from build123d import *

# Parameters (mm, degrees)
IZIM1_W                     = 300
IZIM1_H                     = 120
Y_KSEKLIK_EKSTR_ZYON1_DEPTH = 20
IZIM2_W                     = 20
IZIM2_H                     = 120
Y_KSEKLIK_EKSTR_ZYON2_DEPTH = 70
IZIM3_W                     = 140
IZIM3_H                     = 120
Y_KSEKLIK_EKSTR_ZYON3_DEPTH = 20
Y_KSEKLIK_EKSTR_ZYON4_DEPTH = 20
AYNALAMA3_COPY_1_DEPTH      = 20
IZIM5_R                     = 35
KES_EKSTR_ZYON1_DEPTH       = 51
KES_EKSTR_ZYON1_DEPTH_BACK  = 41
IZIM6_R                     = 10
KES_EKSTR_ZYON2_DEPTH       = 20


with BuildPart() as part:
    # Çizim1 → Yükseklik-Ekstrüzyon1 (new body)
    with BuildSketch(Plane(origin=(0, 0, 0), x_dir=(1, 0, 0), z_dir=(0, 1, 0))):
        with Locations((150, 60)):
            Rectangle(IZIM1_W, IZIM1_H)
    extrude(amount=Y_KSEKLIK_EKSTR_ZYON1_DEPTH)

    # Çizim2 → Yükseklik-Ekstrüzyon2 (add)
    with BuildSketch(Plane(origin=(0, 20, 0), x_dir=(1, 0, 0), z_dir=(0, 1, 0))):
        with Locations((70, 60)):
            Rectangle(IZIM2_W, IZIM2_H)
    y_kseklik_ekstr_zyon2 = extrude(amount=Y_KSEKLIK_EKSTR_ZYON2_DEPTH)

    # Aynalama1: Yükseklik-Ekstrüzyon2 across plane
    add(y_kseklik_ekstr_zyon2.mirror(Plane.ZY.offset(-150)))

    # Çizim3 → Yükseklik-Ekstrüzyon3 (add)
    with BuildSketch(Plane(origin=(0, 20, 0), x_dir=(1, 0, 0), z_dir=(0, 1, 0))):
        with Locations((150, 60)):
            Rectangle(IZIM3_W, IZIM3_H)
    extrude(amount=Y_KSEKLIK_EKSTR_ZYON3_DEPTH)

    # Çizim4 → Yükseklik-Ekstrüzyon4 (add)
    with BuildSketch(Plane.XY):
        Polygon((0, 20), (60, 90), (60, 20), align=None)
    y_kseklik_ekstr_zyon4 = extrude(amount=-Y_KSEKLIK_EKSTR_ZYON4_DEPTH)

    # Aynalama2: Yükseklik-Ekstrüzyon4 across plane
    add(y_kseklik_ekstr_zyon4.mirror(Plane.XY.offset(-60)))

    # Aynalama3: Yükseklik-Ekstrüzyon4 across plane
    add(y_kseklik_ekstr_zyon4.mirror(Plane.ZY.offset(-150)))

    # Aynalama3 copy 1 sketch → Aynalama3 copy 1 (add)
    with BuildSketch(Plane(origin=(300, 0, -120), x_dir=(-1, 0, 0), z_dir=(0, 0, -1))):
        Polygon((0, 20), (60, 90), (60, 20), align=None)
    extrude(amount=-AYNALAMA3_COPY_1_DEPTH)

    # Çizim5 → Kes-Ekstrüzyon1 (cut, two sides)
    with BuildSketch(Plane(origin=(0, 40, 0), x_dir=(1, 0, 0), z_dir=(0, 1, 0))) as kes_ekstr_zyon1_sk:
        with Locations((150, 60)):
            Circle(IZIM5_R)
    extrude(amount=KES_EKSTR_ZYON1_DEPTH, mode=Mode.SUBTRACT)
    extrude(kes_ekstr_zyon1_sk.sketch, amount=-KES_EKSTR_ZYON1_DEPTH_BACK, mode=Mode.SUBTRACT)

    # Çizim6 → Kes-Ekstrüzyon2 (cut)
    with BuildSketch(Plane(origin=(0, 20, 0), x_dir=(1, 0, 0), z_dir=(0, 1, 0))):
        with Locations((25, 60)):
            Circle(IZIM6_R)
        with Locations((275, 60)):
            Circle(IZIM6_R)
    extrude(amount=-KES_EKSTR_ZYON2_DEPTH, mode=Mode.SUBTRACT)


solid = part.part
Verification items for the finished model (mm, model axes). A direction names the side the tool comes from. Coordinates: 2 decimals unless noted, no trailing zeros. Write each loop counter-clockwise with the first axis right and the second up, starting at its lowest first coordinate (ties: lowest second). Pieces come first, ordered by that corner, then holes. Notation, with made-up numbers: (87, -34) - (101, -34) arc R24 ccw to (101, -19) - close; hole circle Ø7 at (72.25, 33.5). An arc over 180 degrees is marked (long way). Answer as a JSON object with one key per item and string values.
(1) Tool access check on faces 1 (the flat face through (220, 65, -59)), 2 (the flat face through (36, 20, -61)), 3 (the flat face through (263, 20, -61)). Record the directions out of +Z, -Z, +X, -X, +Y, -Y that give a thin tool (end or side, any length) a straight path to the whole face; none if there is none.
Report:
{"face 1": "+Z, -Z, +Y", "face 2": "-X, +Y", "face 3": "+X, +Y"}
(2) Gauge pin test, flat ends, axial feed: pin 1 Ø5 at (x, z) = (212, -13.5) entering from +Y; pin 2 Ø21 at (y, z) = (66, -74) entering from +X; pin 3 Ø25 at (y, z) = (55, -55) entering from -X. Record the tip position at first contact, or that the pin passes through.
Report:
{"pin 1": "y = 40", "pin 2": "x = 240", "pin 3": "x = 60"}
(3) Cross-section at D-D on y = 12. Record the cut outline in (x, z).
Report:
{"outline": "(0, -120) - (300, -120) - (300, 0) - (0, 0) - close; hole circle Ø20 at (25, -60); hole circle Ø70 at (150, -60); hole circle Ø20 at (275, -60)"}
(4) Thickness scan on line 1 along X through (y, z) = (8, -60); line 2 along Z through (x, y) = (25, 10.75); line 3 along X through (y, z) = (18.5, -64.5). Record the ranges inside material, lowest first.
Report:
{"line 1": "0 to 15, 35 to 115, 185 to 265, 285 to 300", "line 2": "-120 to -70, -50 to 0", "line 3": "0 to 16.07, 33.93 to 115.29, 184.71 to 266.07, 283.93 to 300"}
(5) Cross-section at A-A on x = 150. Record the cut outline in (y, z).
Report:
{"outline": "(0, -120) - (40, -120) - (40, -95) - (0, -95) - close; (0, -25) - (40, -25) - (40, 0) - (0, 0) - close"}
(6) Mould release check, pull along X, two halves, no side actions. Record for faces 4 (the flat face through (60, 55, -59)), 5 (the flat face through (149, 40, -101)), 6 (the flat face through (230, 90, -61)): pulls with the +X half, pulls with the -X half, needs draft (parallel to the pull), parting line crosses it, or undercut.
Report:
{"face 4": "pulls with the -X half", "face 5": "undercut", "face 6": "needs draft"}
(7) Cross-section at B-B on z = -60. Record the cut outline in (x, y).
Report:
{"outline": "(0, 0) - (15, 0) - (15, 20) - (0, 20) - close; (35, 0) - (115, 0) - (115, 40) - (80, 40) - (80, 90) - (60, 90) - (60, 20) - (35, 20) - close; (185, 0) - (265, 0) - (265, 20) - (240, 20) - (240, 90) - (220, 90) - (220, 40) - (185, 40) - close; (285, 0) - (300, 0) - (300, 20) - (285, 20) - close"}
(8) Cross-section at C-C on y = 58. Record the cut outline in (x, z), plus the area to 3 significant figures.
Report:
{"outline": "(32.57, -120) - (80, -120) - (80, 0) - (32.57, 0) - (32.57, -20) - (60, -20) - (60, -100) - (32.57, -100) - close; (220, -120) - (267.43, -120) - (267.43, -100) - (240, -100) - (240, -20) - (267.43, -20) - (267.43, 0) - (220, 0) - close", "area": "6,990 mm^2"}
